The figure shows three views and two pictorial views of one solid part (mm, origin at its lowest corner). Answer the questions. A direction names the side the tool comes from. Give positions to 0.01 mm unless a question says otherwise; leave off trailing zeros. Write each loop counter-clockwise with the first axis right and the second up, starting at its lowest first coordinate (ties: lowest second). Pieces come first, ordered by that corner, then holes. Notation, with made-up numbers: (55.5, 12) -> (65.5, 12) arc R24 cw to (65.5, 31) -> close; hole circle Ø2 at (-18, -27.75). An arc over 180 degrees is marked (long way). Write each question's results on one line, items separated by ' | '. Start each with the question number.
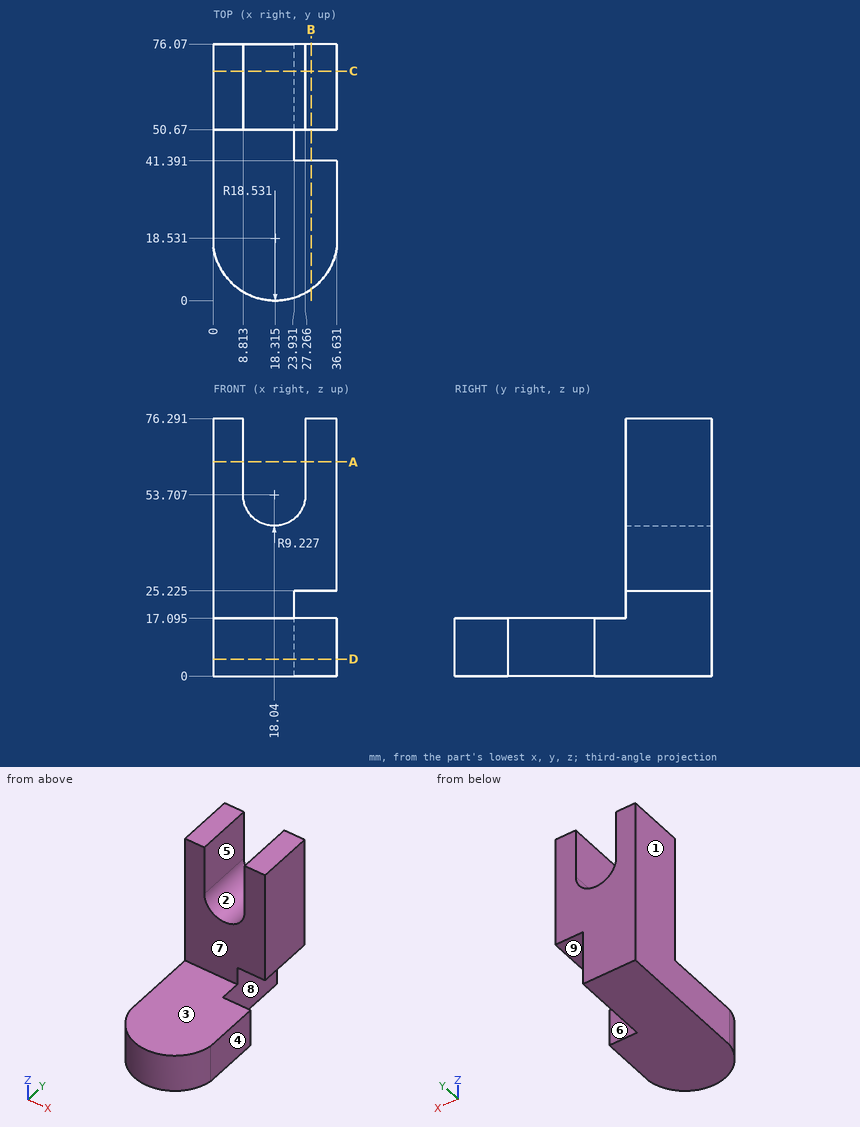
1. Each of these flat-tipped pins is pushed along its axis until it touches: pin 1 Ø18.5 at (x, z) = (13.5, 55) entering from -Y; pin 2 Ø10 at (x, z) = (29, 9) entering from +Y; pin 3 Ø12.5 at (y, z) = (66, 12) entering from +X. Where does it stop, or does it pass through?
2. The mould has two halves that part along X. Classify the marked faces 1, 2, 3 and 4: pulls with the +X half, pulls with the -X half, needs draft (parallel to the pull), parting line crosses it, or undercut.
3. Section D-D (z = 5) is taken. Write down the section's boundary in (x, y) (1 decimal), then the cut area to 3 significant figures.
4. A tool of negligible diameter and unlimited length cuts with its end or side. For the marked faces 5, 6, 7, 8 and 9, from which of +Z, -Z, +X, -X, +Y, -Y can it reach the whole face along a straight path? Write none if from no direction.
5. Section B-B (x = 29) is taken. Write down the section's boundary in (y, z) (1 decimal).
6. Section C-C (y = 68) is taken. Write down the section's boundary in (x, z) (1 decimal), then the cut area to 3 significant figures.
7. Section A-A (z = 63.5) is taken. Write down the section's boundary in (x, y).
8. Consider probe 1 along X at (y, z) = (51.5, 54); probe 2 along Z at (x, y) = (17, 33) (1 decimal); probe 3 along Y at (x, z) = (16.5, 37.5). Determine where each line is inside the solid, lowest interval first. Write a range as [from, to].
Results:
1) pin 1: stops at y = 50.67 | pin 2: stops at y = 41.39 | pin 3: stops at x = 23.93
2) face 1: pulls with the -X half | face 2: undercut | face 3: needs draft | face 4: pulls with the +X half
3) outline: (0, 15.7) arc R18.5 ccw to (36.6, 15.7) -> (36.6, 41.4) -> (23.9, 41.4) -> (23.9, 76.1) -> (0, 76.1) -> close | area: 2,210 mm²
4) face 5: +Z, +Y, -Y | face 6: +Z, -Z, +X, +Y | face 7: +Z, +X, -X, -Y | face 8: -Z, +X, +Y | face 9: -Z, +X, +Y, -Y
5) outline: (3.4, 0) -> (41.4, 0) -> (41.4, 17.1) -> (3.4, 17.1) -> close; (50.7, 25.2) -> (76.1, 25.2) -> (76.1, 76.3) -> (50.7, 76.3) -> close
6) outline: (0, 0) -> (23.9, 0) -> (23.9, 25.2) -> (36.6, 25.2) -> (36.6, 76.3) -> (27.3, 76.3) -> (27.3, 53.7) arc R9.2 cw to (8.8, 53.7) -> (8.8, 76.3) -> (0, 76.3) -> close | area: 1,920 mm²
7) outline: (0, 50.67) -> (8.81, 50.67) -> (8.81, 76.07) -> (0, 76.07) -> close; (27.27, 50.67) -> (36.63, 50.67) -> (36.63, 76.07) -> (27.27, 76.07) -> close
8) probe 1: x = [0, 8.81], [27.27, 36.63] | probe 2: z = [0, 17.1] | probe 3: y = [50.67, 76.07]
